from build123d import *

# Parameters (mm, degrees)
F0_W        = 127
F0_H        = 254
F1_DEPTH    = 2.54
F2_W        = 12.7
F2_H        = 25.4
F3_DEPTH    = 12.7
F4_W        = 6.35
F4_H        = 12.7
F5_DEPTH    = 25.4
F6_T1_DEPTH = 12.7


# Not quite as in the source:
# - a fillet or chamfer that OpenCascade refuses, or shapes differently, is made with other operations: its cross-section is extruded or revolved along the edge and cut away or added


with BuildPart() as f1:
    # F0 (on Front) → F1 (new body, symmetric)
    with BuildSketch(Plane.XZ):
        with Locations((0, -5.0209306781)):
            Rectangle(F0_W, F0_H)
    extrude(amount=F1_DEPTH, both=True)

    # F2 (on face) → F3 (join)
    with BuildSketch(Plane.XZ.offset(2.54)):
        with Locations((-44.3181917071, 0)):
            Rectangle(F2_W, F2_H)
    extrude(amount=F3_DEPTH)

    # F4 (on face) → F5 (cut)
    with BuildSketch(Plane(origin=(-50.6681917071, 0, 0), x_dir=(0, -1, 0), z_dir=(-1, 0, 0))):
        with Locations((8.9468448423, -0.4299022911)):
            Rectangle(F4_W, F4_H)
    extrude(amount=-F5_DEPTH, mode=Mode.SUBTRACT)

    # F6: fillet of radius 5.08 on 2 edges, made by hand

    # F6_s2 → F6_t1 (cut)
    with BuildSketch(Plane.XY.offset(-6.7799022911)):
        with BuildLine():
            ThreePointArc((-50.6681917071, -17.2018448423), (-49.1802941556, -13.6097423939), (-45.5881917071, -12.1218448423))
            Line((-45.5881917071, -12.1218448423), (-50.6681917071, -12.1218448423))
            Line((-50.6681917071, -12.1218448423), (-50.6681917071, -17.2018448423))
        make_face()
        with BuildLine():
            ThreePointArc((-37.9681917071, -17.2018448423), (-39.4560892587, -13.6097423939), (-43.0481917071, -12.1218448423))
            Line((-43.0481917071, -12.1218448423), (-37.9681917071, -12.1218448423))
            Line((-37.9681917071, -12.1218448423), (-37.9681917071, -17.2018448423))
        make_face()
    extrude(amount=F6_T1_DEPTH, mode=Mode.SUBTRACT)


solid = f1.part
Source: CAD feature listing. Evaluate the final solid. Frame: model axes, mm. A direction names the side the tool comes from. Round coordinates to 2 decimals unless told otherwise and drop trailing zeros. Loops run counter-clockwise (first coordinate to the right, second up) from the corner with the lowest first, then second, coordinate; pieces in that order, holes last. Notation, with made-up numbers: (8.25, 69) -> (56.25, 69) arc R36 ccw to (56.25, 104) -> close; hole circle Ø3 at (42, -36.5). An arc over 180 degrees is marked (long way). Answer as a JSON object with one key per item and string values. Group by question number.
Q1. Section query C-C (x = -15). Output: boundary loops of the cut face in (y, z), plus the area to 3 significant figures.
Q2. Section query A-A (y = -8.75). Output: boundary loops of the cut face in (x, z), plus the area to 3 significant figures.
Q3. Ray query, line 1 (Y direction, x = -24, z = 30.5). Return the intervals inside material, ascending. Write a range as from..to.
Q4. Contact query for flat-ended pins moving along their axis: P1, Ø4, axis at y = -10.5, z = -5, coming from the -X side; P2, Ø10, axis at x = -45, y = -8, coming from the -Z side; P3, Ø4, axis at x = -47, y = -6, coming from the +Z side; P4, Ø8, axis at x = 12, y = -8, coming from the +Z side. Output: stop coordinate, or through.
Q5. Section query B-B (z = 99.5). Output: boundary loops of the cut face in (x, y).
Q6. Mould query, pull axis Y, two halves, no side actions, for faces 5 (the cylindrical face through (-40.199, -12.996, -0.519)), 6 (the flat face through (-1, 2.54, -3)), 7 (the flat face through (-44, -9, 5.92)), 8 (the flat face through (-44, -9, 12.7)). Classes: pulls with the +Y half, pulls with the -Y half, needs draft (parallel to the pull), parting line crosses it, or undercut.
Q7. Access query for faces 1 (the cylindrical face through (-48.44, -13, -0.52)), 2 (the flat face through (-44, -5.772, -1)), 3 (the flat face through (-44, -9, -12.7)), 4 (the flat face through (-50.668, -5, 0)). Directions: +Z, -Z, +X, -X, +Y, -Y. A direction counts if a zero-diameter tool reaches every point of the face in a straight line with its end or side. Return the directions, or none.
Completed:
{
 "1": {"outline": "(-2.54, -132.02) -> (2.54, -132.02) -> (2.54, 121.98) -> (-2.54, 121.98) -> close", "area": "1,290 mm²"},
 "2": {"outline": "(-50.67, -12.7) -> (-37.97, -12.7) -> (-37.97, -6.78) -> (-50.67, -6.78) -> close; (-50.67, 5.92) -> (-37.97, 5.92) -> (-37.97, 12.7) -> (-50.67, 12.7) -> close", "area": "161 mm²"},
 "3": {"line 1": "-2.54..2.54"},
 "4": {"P1": "x = -50.67", "P2": "z = -12.7", "P3": "z = 12.7", "P4": "through"},
 "5": {"outline": "(-63.5, -2.54) -> (63.5, -2.54) -> (63.5, 2.54) -> (-63.5, 2.54) -> close"},
 "6": {"face 5": "undercut", "face 6": "pulls with the +Y half", "face 7": "undercut", "face 8": "needs draft"},
 "7": {"face 1": "-X", "face 2": "+X, -X", "face 3": "-Z, +X, -X, -Y", "face 4": "+Z, -Z, -X, -Y"}
}
